Autodesk Inventor part; units mm, degrees
ref_plane "YZ Plane" through (0, 0, 0) normal (1, 0, 0) x (0, 1, 0)
ref_plane "XZ Plane" through (0, 0, 0) normal (0, 1, 0) x (-1, 0, 0)
ref_plane "XY Plane" through (0, 0, 0) normal (0, 0, 1) x (1, 0, 0)
sketch "Sketch1" plane through (0, 0, 0) normal (0, 1, 0) x (-1, 0, 0)
  circle A0 centre (0, 0) radius 20
  line L0 (0, 0) -> (0, 7)
  line L1 (0, 0) -> (-7, 0)
  line L2 (0, 0) -> (0, -7)
  line L3 (0, 0) -> (7, 0)
  circle A1 centre (-7, 0) radius 1.5
  circle A2 centre (0, 7) radius 1.5
  circle A3 centre (0, -7) radius 1.5
  circle A4 centre (7, 0) radius 1.5
  dimension "d0" = 40
  dimension "d1" = 7
  dimension "d2" = 7
  dimension "d3" = 7
  dimension "d4" = 7
  dimension "d5" = 3
  dimension "d6" = 3
  dimension "d8" = 3
  dimension "d11" = 3
extrude "Extrusion2" add sketch "Sketch1" along normal blind 3
properties part number "Wrist Sprocket"
Can you work these out from the model? Positions are in its coordinate system, mm. Give positions to 0.01 mm unless a question says otherwise; leave off trailing zeros. Order: outer loops, then holes, each group sorted by start corner. A loop starts at its lowest first (then second) coordinate and runs counter-clockwise, first axis right, second up. Notation, with made-up numbers: M 84,64 L 91,64 A18 ccw 91,72 Z; hole C 59,86 d3. An arc over 180 degrees is marked long. Write item = value, one per line. Start each with the question number.
Q1. Suppose I cut it at B-B (x = 0). Write out the boundary of the cut face in (y, z), plus the area to 3 significant figures.
Q2. Suppose I cut it at A-A (z = 0). Write out the boundary of the cut face in (x, y).
Q3. Suppose I cut it at C-C (x = 7). Write out the boundary of the cut face in (y, z) (3 decimals).
Q4. I need wall thicknesses on probe 1 along Z at (x, y) = (0, 1.95); probe 2 along Z at (x, y) = (-1, 0.55); probe 3 along Z at (x, y) = (-7, 0.9) (3 decimals). Which ranges of each line are inside material? Lowest first, please. Write a range as [from, to].
Q5. We'd pull the mould along X, two halves only. Please class faces 1 (the cylindrical face through (0.325, 1.479, 8.464)), 2 (the cylindrical face through (4.336, 1.479, 19.524)), 3 (the cylindrical face through (0.325, 1.479, -5.536)), 4 (the flat face through (0, 3, 0)): pulls with the +X half, pulls with the -X half, needs draft (parallel to the pull), parting line crosses it, or undercut.
Q6. Will this pin go through, and if not, where does the flat tip stop? pin 1 Ø2.5 at (x, z) = (7, 0) entering from -Y.
Q7. Suppose I cut it at D-D (z = 6). Write out the boundary of the cut face in (x, y), plus the area to 3 significant figures.
Check result:
q1.outline = M 0,-20 L 3,-20 L 3,-8.5 L 0,-8.5 Z; M 0,-5.5 L 3,-5.5 L 3,5.5 L 0,5.5 Z; M 0,8.5 L 3,8.5 L 3,20 L 0,20 Z
q1.area = 102 mm2
q2.outline = M -20,0 L -8.5,0 L -8.5,3 L -20,3 Z; M -5.5,0 L 5.5,0 L 5.5,3 L -5.5,3 Z; M 8.5,0 L 20,0 L 20,3 L 8.5,3 Z
q3.outline = M 0,-18.735 L 3,-18.735 L 3,-1.5 L 0,-1.5 Z; M 0,1.5 L 3,1.5 L 3,18.735 L 0,18.735 Z
q4.probe_1 = [-20, -8.5], [-5.5, 5.5], [8.5, 20]
q4.probe_2 = [-19.97, -8.12], [-5.88, 5.88], [8.12, 19.97]
q4.probe_3 = [-18.735, -1.5], [1.5, 18.735]
q5.face_1 = undercut
q5.face_2 = parting line crosses it
q5.face_3 = undercut
q5.face_4 = needs draft
q6.pin_1 = through
q7.outline = M -19.08,0 L -1.12,0 L -1.12,3 L -19.08,3 Z; M 1.12,0 L 19.08,0 L 19.08,3 L 1.12,3 Z
q7.area = 108 mm2
